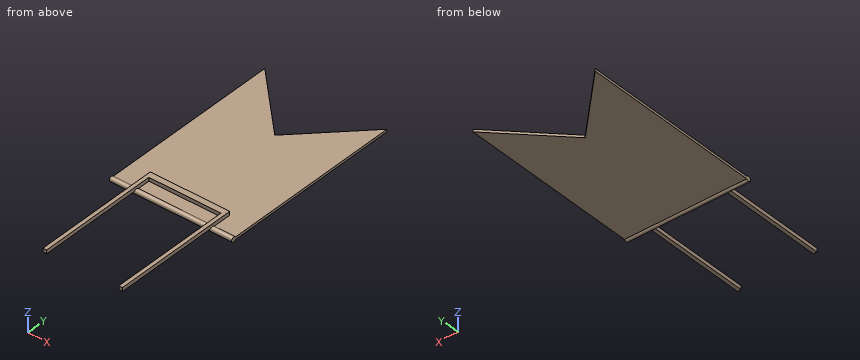
Autodesk Inventor part; units mm, degrees
ref_plane "YZ Plane" through (0, 0, 0) normal (1, 0, 0) x (0, 1, 0)
ref_plane "XZ Plane" through (0, 0, 0) normal (0, 1, 0) x (-1, 0, 0)
ref_plane "XY Plane" through (0, 0, 0) normal (0, 0, 1) x (1, 0, 0)
sketch "草圖1" plane through (0, 0, 0) normal (0, 0, 1) x (1, 0, 0)
  line L0 (-500, -500) -> (0, -1000)
  line L1 (0, -1000) -> (500, -500)
  line L2 (-500, -500) -> (-500, -2000)
  line L3 (-500, -2000) -> (500, -2000)
  line L4 (500, -2000) -> (500, -500)
  point P0 (0, 0)
  dimension "d2" = 1500
  dimension "d3" = 1000
extrude "擠出1" add sketch "草圖1" along normal blind 20
sketch "草圖2" plane through (500, -2000, 0) normal (1, 0, 0) x (0, 0, -1)
  line L0 (0, 0) -> (-20, 0)
  circle A0 centre (-10, 0) radius 20
  point P0 (0, 2000)
  dimension "d6" = 40
extrude "擠出2" add sketch "草圖2" against normal blind 1000
sketch "草圖3" plane through (0, 0, 20) normal (0, 0, 1) x (1, 0, 0)
  line L0 (325, -1879.5485) -> (-325, -1879.5485)
  line L1 (-325, -1879.5485) -> (-325, -1829.5485)
  line L2 (-325, -1829.5485) -> (325, -1829.5485)
  line L3 (325, -1829.5485) -> (325, -1879.5485)
  line L4 (325, -1879.5485) -> (-325, -1829.5485) construction
  line L5 (-325, -1879.5485) -> (325, -1829.5485) construction
  point P0 (0, 0)
  point P1 (0, -1854.5485)
  dimension "d9" = 650
  dimension "d10" = 50
extrude "擠出3" add sketch "草圖3" along normal blind 30
sketch "草圖4" plane through (-325, -1879.5485, 20) normal (0, -1, 0) x (1, 0, 0)
  line L0 (650, 0) -> (0, 0)
  line L1 (0, 30) -> (650, 30)
  line L2 (650, 0) -> (620, 0)
  line L3 (620, 0) -> (620, 30)
  line L4 (620, 30) -> (650, 30)
  line L5 (650, 30) -> (650, 0)
  line L6 (0, 0) -> (650, 0)
  line L7 (0, 30) -> (30, 30)
  line L8 (30, 30) -> (30, 0)
  line L9 (30, 0) -> (0, 0)
  line L10 (0, 0) -> (0, 30)
  point P0 (325, -20)
  dimension "d13" = 30
  dimension "d14" = 30
extrude "擠出4" add sketch "草圖4" along normal blind 1000 contours L0 L3 L1 L5
extrude "擠出5" add sketch "草圖4" along normal blind 1000 contours L0 L10 L1 L8
properties part number "flag"
Can you work these out from the model? Positions are in its coordinate system, mm. Round coordinates to 2 decimals unless told otherwise and drop trailing zeros. Write each loop counter-clockwise with the first axis right and the second up, starting at its lowest first coordinate (ties: lowest second). Pieces come first, ordered by that corner, then holes. Notation, with made-up numbers: M 25,80.25 L 45,80.25 A12 ccw 45,85.25 Z; hole C 84,14.5 d3. An arc over 180 degrees is marked long. Use a Markdown table: item, result.
Item 1: For pin 1 Ø24 at (y, z) = (-2199.5, 34.5) entering from -X; pin 2 Ø9 at (x, z) = (67, 36) entering from -Y; pin 3 Ø24 at (x, z) = (-144, 39) entering from +Y; pin 4 Ø12 at (y, z) = (-799, -2) entering from -X, each with a flat end and sliding along its axis, tell me the tip position at first contact or that it passes through.
Found:
| item | result |
|---|---|
| pin 1 | stops at x = -325 |
| pin 2 | stops at y = -1879.55 |
| pin 3 | stops at y = -1829.55 |
| pin 4 | stops at x = -500 |
Item 2: I want a section at C-C (x = 417). List the corners of the cut face in (y, z) for me, and give its area (3 significant figures).
Found:
| item | result |
|---|---|
| outline | M -1982.68,0 L -583,0 L -583,20 L -1982.68,20 A20 ccw long Z |
| area | 29,200 mm2 |
Item 3: I want a section at A-A (y = -722.5). List the corners of the cut face in (x, z) for me.
Found:
| item | result |
|---|---|
| outline | M -500,0 L -277.5,0 L -277.5,20 L -500,20 Z; M 277.5,0 L 500,0 L 500,20 L 277.5,20 Z |
Item 4: If I drill on line 1 along X through (y, z) = (-2152.5, 27); line 2 along X through (y, z) = (-997, 2.5); line 3 along Z through (x, y) = (-55, -1725.5), over which ranges is the centre line in solid material (lowest first)? Write a range as [from, to].
Found:
| item | result |
|---|---|
| line 1 | x = [-325, -295], [295, 325] |
| line 2 | x = [-500, -3], [3, 500] |
| line 3 | z = [0, 20] |
Item 5: I want a section at D-D (y = -2630). List the corners of the cut face in (x, z) for me.
Found:
| item | result |
|---|---|
| outline | M -325,20 L -295,20 L -295,50 L -325,50 Z; M 295,20 L 325,20 L 325,50 L 295,50 Z |
Item 6: I want a section at B-B (z = 10). List the corners of the cut face in (x, y) for me, and give its area (3 significant figures).
Found:
| item | result |
|---|---|
| outline | M -500,-2020 L 500,-2020 L 500,-500 L 0,-1000 L -500,-500 Z |
| area | 1,270,000 mm2 |
